Autodesk Inventor part; units mm, degrees
ref_plane "YZ Plane" through (0, 0, 0) normal (1, 0, 0) x (0, 1, 0)
ref_plane "XZ Plane" through (0, 0, 0) normal (0, 1, 0) x (-1, 0, 0)
ref_plane "XY Plane" through (0, 0, 0) normal (0, 0, 1) x (1, 0, 0)
sketch "Sketch1" plane through (0, 0, 0) normal (0, 0, 1) x (1, 0, 0)
  line L0 (-48, 48) -> (48, 48)
  line L1 (48, 48) -> (48, -48)
  line L2 (48, -48) -> (-48, -48)
  line L3 (-48, -48) -> (-48, 48)
  line L4 (38, 38) -> (-38, 38)
  line L5 (-38, 38) -> (-38, -38)
  line L6 (-38, -38) -> (38, -38)
  line L7 (38, -38) -> (38, 38)
  line L8 (0, 61.066) -> (0, -72.1628) construction
  line L9 (-77.8847, 0) -> (88.8171, 0) construction
  line L10 (-48, 43) -> (48, 43) construction
  line L11 (-43, 48) -> (-43, -48) construction
  line L12 (-48, -43) -> (48, -43) construction
  circle A0 centre (-43, 25) radius 2.25
  circle A1 centre (-43, -25) radius 2.25
  circle A2 centre (-43, -43) radius 2.25
  circle A3 centre (-43, 43) radius 2.25
  line L13 (-48, 30) -> (48, 30) construction
  line L14 (-48, -30) -> (48, -30) construction
  line L15 (-50, 31) -> (-36, 31)
  line L16 (-36, 31) -> (-36, -31)
  line L17 (-36, -31) -> (-50, -31)
  line L18 (-50, -31) -> (-50, 31)
  point P0 (0, 0)
  point P1 (0, 48)
  point P2 (48, 0)
  dimension "d0" = 96
  dimension "d1" = 96
  dimension "d2" = 10
  dimension "d5" = 5
  dimension "d11" = 5
  dimension "d14" = 5
  dimension "d31" = 4.5
  dimension "d32" = 4.5
  dimension "d61" = 4.5
  dimension "d62" = 4.5
  dimension "d65" = 30
  dimension "d66" = 30
  dimension "d67" = 5
  dimension "d68" = 5
  dimension "d74" = 1
  dimension "d75" = 1
  dimension "d76" = 2
  dimension "d77" = 2
extrude "Extrusion1" add sketch "Sketch1" against normal blind 1.5 contours L0 L1 L2 L3 L17 L5 L6 L7 L4 L15 | L15 L5 L17 L3 | A0 | A1 | A2 | A3
extrude "Extrusion2" cut sketch "Sketch1" against normal blind 10 contours A2 | A3
mirror "Mirror5" about plane through (0, 0, 0) normal (1, 0, 0) of "Extrusion2"
extrude "Extrusion5" cut sketch "Sketch1" against normal blind 10 contours A0 | A1
pattern_circular "Circular Pattern2" count 4 over 360 about axis through (0, 0, -10) along (0, 0, 1) of "Extrusion5"
sketch "Sketch5" plane through (0, 0, 0) normal (0, 0, 1) x (1, 0, 0)
  line L0 (-48, -48) -> (-48, 48)
  line L1 (-38, -38) -> (-38, 38)
  line L2 (-48, -35.5) -> (-38, -35.5)
  line L3 (-38, -35.5) -> (-38, -32.5)
  line L4 (-38, -32.5) -> (-48, -32.5)
  line L5 (-48, -32.5) -> (-48, -35.5)
  line L6 (-51.6876, -22.75) -> (-34.0834, -22.75)
  line L7 (-34.0834, -22.75) -> (-34.0834, -45.25)
  line L8 (-34.0834, -45.25) -> (-51.6876, -45.25)
  line L9 (-51.6876, -45.25) -> (-51.6876, -22.75)
  circle A0 centre (-43, -25) radius 2.25
  circle A1 centre (-43, -43) radius 2.25
  line L10 (-22.75, -50) -> (-45.25, -50)
  line L11 (-45.25, -50) -> (-45.25, -36.2343)
  line L12 (-45.25, -36.2343) -> (-22.75, -36.2343)
  line L13 (-22.75, -36.2343) -> (-22.75, -50)
  circle A2 centre (-25, -43) radius 2.25
  line L14 (38, -38) -> (-38, -38)
  line L15 (48, -48) -> (-48, -48)
  line L16 (-32.5, -38) -> (-35.5, -38)
  line L17 (-35.5, -38) -> (-35.5, -48)
  line L18 (-35.5, -48) -> (-32.5, -48)
  line L19 (-32.5, -48) -> (-32.5, -38)
  line L20 (-32.5, -32.5) -> (-38, -32.5)
  line L21 (-38, -32.5) -> (-38, -35.5)
  line L22 (-38, -35.5) -> (-32.5, -35.5)
  line L23 (-32.5, -35.5) -> (-32.5, -32.5)
  line L24 (-32.5, -35.5) -> (-35.5, -35.5)
  line L25 (-35.5, -35.5) -> (-35.5, -38)
  line L26 (-35.5, -38) -> (-32.5, -38)
  line L27 (-32.5, -38) -> (-32.5, -35.5)
  line L28 (-38, -38) -> (-35.5, -38)
  line L29 (-35.5, -38) -> (-35.5, -35.5)
  line L30 (-35.5, -35.5) -> (-38, -35.5)
  line L31 (-38, -35.5) -> (-38, -38)
  point P0 (0, 0)
  point P1 (-38, -34)
  point P2 (-34.0834, -34)
  point P3 (-34, -38)
  point P4 (-34, -36.2343)
  dimension "d95" = 3
  dimension "d96" = 3
extrude "Extrusion9" add sketch "Sketch5" along normal blind 15 contours L0 L4 L1 L2 | L1 L20 L7 L22 | L22 L7 L12 L25 | L20 L23 L22 L7 | L12 L7 L14 L25 | L22 L27 L12 L7 | L17 L8 L7 L14 L19 L15 | L17 L14 L7 L8 | L12 L27 L14 L7
extrude "Extrusion10" add sketch "Sketch5" against normal blind 1.5 contours L22 L25 L12 L1 | L1 L20 L7 L22 | L12 L25 L14 L1 | L22 L7 L12 L25 | L20 L23 L22 L7 | L12 L7 L14 L25 | L22 L27 L12 L7 | L12 L27 L14 L7
sketch "Sketch6" plane through (-48, -35.5, 15) normal (0, -1, 0) x (1, 0, 0)
  line L0 (12.5, -15) -> (12.5, 0)
  line L1 (0, 0) -> (12.5, 0)
  line L2 (0, -15) -> (0, 0)
  line L3 (0, -15) -> (12.5, -15)
  circle A0 centre (6.25, -4) radius 2.25
  point P0 (48, -15)
  dimension "d101" = 4.5
  dimension "d102" = 4
extrude "Extrusion11" cut sketch "Sketch6" against normal blind 5 contours A0
sketch "Sketch7" plane through (-35.5, -48, 0) normal (-1, 0, 0) x (0, 0, 1)
  line L0 (0, 12.5) -> (0, 0)
  line L1 (0, 0) -> (15, 0)
  line L2 (15, 12.5) -> (15, 0)
  line L3 (0, 12.5) -> (15, 12.5)
  circle A0 centre (11, 6.25) radius 2.25
  point P0 (0, 48)
  dimension "d105" = 4.5
  dimension "d106" = 4
extrude "Extrusion12" cut sketch "Sketch7" against normal blind 5 contours A0
pattern_circular "Circular Pattern3" count 4 over 360 about axis through (0, 0, -10) along (0, 0, 1) of "Extrusion9", "Extrusion10", "Extrusion11", "Extrusion12"
sketch "Sketch8" plane through (0, 0, 0) normal (0, 0, 1) x (1, 0, 0)
  line L0 (48, 48) -> (48, -48)
  line L1 (-48, 48) -> (48, 48)
  line L2 (-48, 35.5) -> (-48, 48)
  line L3 (-48, -48) -> (-48, 48)
  line L4 (48, -48) -> (-48, -48)
  circle A0 centre (0, 0) radius 7.5
  circle A1 centre (0, 0) radius 12.5
  line L5 (-40.4749, -35.5251) -> (35.5251, 40.4749)
  line L6 (35.5251, 40.4749) -> (40.4749, 35.5251)
  line L7 (40.4749, 35.5251) -> (-35.5251, -40.4749)
  line L8 (-35.5251, -40.4749) -> (-40.4749, -35.5251)
  line L9 (-38, -38) -> (38, 38) construction
  line L10 (-2.4749, 2.4749) -> (2.4749, -2.4749) construction
  line L11 (-32.5, 38) -> (32.5, 38)
  line L12 (38, 38) -> (-38, 38)
  line L13 (38, -38) -> (38, 38)
  dimension "d112" = 15
  dimension "d113" = 5
  dimension "d114" = 7
extrude "Extrusion13" add sketch "Sketch8" against normal blind 1.5 contours A0 L7 A1 | A0 L5 A1 L7 | L7 A1 L5 A0 | A0 L5 A1
extrude "Extrusion14" add sketch "Sketch8" against normal blind 1.5 contours L7 A0 L5 | A0 L5 A1 L7 | L7 A1 L5 A0 | A1 L5 L12 L13 L7 | L7 L8 L5 A1 | L13 L6 L7 | L5 L6 L12
mirror "Mirror8" about plane through (0, 0, 0) normal (0, 1, 0) of "Extrusion14"
extrude "Extrusion15" cut sketch "Sketch8" against normal blind 1.5 contours A0 L7 | L7 A0 L5 | L5 A0
equation "\"d31\" = screw"
equation "\"d32\" = screw"
equation "\"d61\" = screw"
equation "\"d62\" = screw"
equation "\"d101\" = screw"
equation "\"d105\" = screw"
properties part number "Base" material "PC/ABS Plastic"
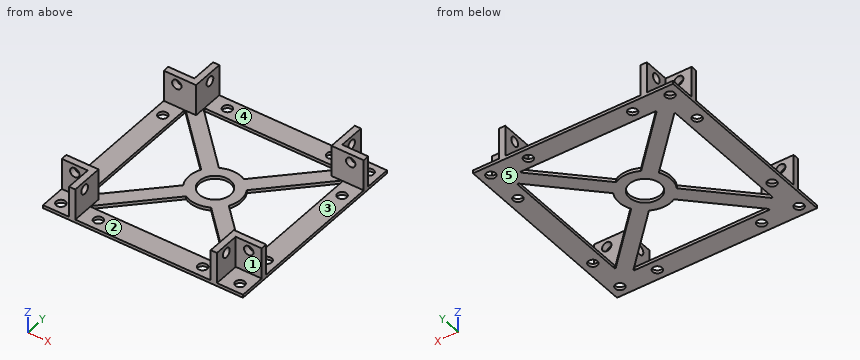
CAD build for the part. Positions are in the model's coordinates, mm. Face numbers are marked on the shaded views. A direction names the side the tool comes from. Coordinates: 2 decimals unless noted, no trailing zeros. Write each loop counter-clockwise with the first axis right and the second up, starting at its lowest first coordinate (ties: lowest second). Pieces come first, ordered by that corner, then holes. Notation, with made-up numbers: M 37.25,71 L 50.25,71 A17 cw 50.25,102 Z; hole C 8,8 d8. An arc over 180 degrees is marked long. Answer as a JSON object with one key per item and string values. Group by question number.
1) Wall check: line 1 (Y direction, x = 43, z = -0.6); line 2 (Y direction, x = 35, z = 2.75); line 3 (Y direction, x = 41, z = 13.5). Give the ranges that are in metal, low to high. Write a range as from..to.
2) Saw through at D-D (x = -9). Write the cut outline in (y, z).
3) Saw through at C-C (x = 20.5). Write the cut outline in (y, z), plus the area to 3 significant figures.
4) Pin check, flat tips, straight feed: pin 1 Ø5 at (x, y) = (-43, -43) entering from +Z; pin 2 Ø4.5 at (x, z) = (-40.5, 3) entering from -Y; pin 3 Ø6 at (x, z) = (-41.75, 11) entering from +Y. Stop position of each tip, or through.
5) Tool access for the marked faces 1, 2 and 3: list every direction of +Z, -Z, +X, -X, +Y, -Y with a clear straight run to the whole face (end or side of a thin tool).
6) Mould opens along X. For the marked faces 4 and 5 say: +X half, -X half, draft (parallel to the pull), parting line (faces both ways), or undercut.
7) Saw through at B-B (y = -31). Write the cut outline in (x, z), plus the area to 3 significant figures.
8) Saw through at A-A (z = 7.25). Write the cut outline in (x, y), plus the area to 3 significant figures.
Values follow:
{
 "1": {"line 1": "y = -48..-45.25, -40.75..-27.25, -22.75..22.75, 27.25..40.75, 45.25..48", "line 2": "y = -48..-32.5, 32.5..48", "line 3": "y = -35.5..-32.5, 32.5..35.5"},
 "2": {"outline": "M -48,-1.5 L -38,-1.5 L -38,0 L -48,0 Z; M -13.95,-1.5 L 13.95,-1.5 L 13.95,0 L -13.95,0 Z; M 38,-1.5 L 48,-1.5 L 48,0 L 38,0 Z"},
 "3": {"outline": "M -48,-1.5 L -38,-1.5 L -38,0 L -48,0 Z; M -25.45,-1.5 L -15.55,-1.5 L -15.55,0 L -25.45,0 Z; M 15.55,-1.5 L 25.45,-1.5 L 25.45,0 L 15.55,0 Z; M 38,-1.5 L 48,-1.5 L 48,0 L 38,0 Z", "area": "59.7 mm2"},
 "4": {"pin 1": "stops at z = 0", "pin 2": "stops at y = -35.5", "pin 3": "stops at y = 35.5"},
 "5": {"face 1": "+Z, +X, -Y", "face 2": "+Z, +Y, -Y", "face 3": "+Z, +X, -X"},
 "6": {"face 4": "undercut", "face 5": "draft"},
 "7": {"outline": "M -48,-1.5 L -38,-1.5 L -38,0 L -48,0 Z; M -35.95,-1.5 L -26.05,-1.5 L -26.05,0 L -35.95,0 Z; M 26.05,-1.5 L 35.95,-1.5 L 35.95,0 L 26.05,0 Z; M 38,-1.5 L 48,-1.5 L 48,0 L 38,0 Z", "area": "59.7 mm2"},
 "8": {"outline": "M -48,-35.5 L -35.5,-35.5 L -35.5,-48 L -32.5,-48 L -32.5,-32.5 L -48,-32.5 Z; M -48,32.5 L -32.5,32.5 L -32.5,48 L -35.5,48 L -35.5,35.5 L -48,35.5 Z; M 32.5,-48 L 35.5,-48 L 35.5,-35.5 L 48,-35.5 L 48,-32.5 L 32.5,-32.5 Z; M 32.5,32.5 L 48,32.5 L 48,35.5 L 35.5,35.5 L 35.5,48 L 32.5,48 Z", "area": "336 mm2"}
}
